Autodesk Inventor part; units mm, degrees
ref_plane "YZ Plane" through (0, 0, 0) normal (1, 0, 0) x (0, 1, 0)
ref_plane "XZ Plane" through (0, 0, 0) normal (0, 1, 0) x (-1, 0, 0)
ref_plane "XY Plane" through (0, 0, 0) normal (0, 0, 1) x (1, 0, 0)
sketch "Sketch1" plane through (0, 0, 0) normal (1, 0, 0) x (0, 1, 0)
  line L0 (0, 0) -> (-25.4, 0)
  line L1 (-25.4, 0) -> (-25.4, -25.4)
  line L2 (-25.4, -25.4) -> (0, -25.4)
  line L3 (0, -25.4) -> (0, 0)
  line L4 (-3.175, -22.225) -> (-22.225, -22.225)
  line L5 (-22.225, -22.225) -> (-22.225, -3.175)
  line L6 (-22.225, -3.175) -> (-3.175, -3.175)
  line L7 (-3.175, -3.175) -> (-3.175, -22.225)
  dimension "d0" = 25.4
  dimension "d1" = 25.4
  dimension "d2" = 3.175
extrude "Extrusion1" add sketch "Sketch1" along normal blind 50.8
sketch "Sketch2" plane through (0, -25.4, 0) normal (0, 0, 1) x (1, 0, 0)
  circle A0 centre (25.4, 12.7) radius 4.7625
  line L0 (0, 25.4) -> (50.8, 25.4)
  line L1 (0, 25.4) -> (0, 0)
  dimension "d5" = 9.525
  dimension "d6" = 12.7
  dimension "d7" = 25.4
extrude "Extrusion2" cut sketch "Sketch2" against normal blind 50.8
sketch "Sketch3" plane through (0, 0, 0) normal (0, 1, 0) x (1, 0, 0)
  circle A0 centre (41.275, 12.7) radius 3.175
  circle A1 centre (9.525, 12.7) radius 3.175
  line L0 (50.8, 25.4) -> (50.8, 0)
  line L1 (0, 25.4) -> (50.8, 25.4)
  line L2 (0, 22.225) -> (0, 3.175)
  point P0 (0, 0)
  dimension "d10" = 6.35
  dimension "d11" = 6.35
  dimension "d12" = 9.525
  dimension "d13" = 12.7
  dimension "d14" = 9.525
  dimension "d15" = 12.7
extrude "Extrusion3" cut sketch "Sketch3" against normal blind 3.175
sketch "Sketch4" plane through (0, -25.4, -25.4) normal (0, -1, 0) x (1, 0, 0)
  circle A0 centre (41.275, 12.7) radius 3.175
  circle A1 centre (41.275, 12.7) radius 4.7625
  circle A2 centre (9.525, 12.7) radius 4.7625
  line L0 (0, 25.4) -> (0, 0)
  line L1 (0, 0) -> (50.8, 0)
  dimension "d18" = 9.525
  dimension "d19" = 9.525
  dimension "d20" = 9.525
  dimension "d21" = 12.7
extrude "Extrusion4" cut sketch "Sketch4" against normal blind 3.175 contours A0 | A1 | A2
properties part number "15102898-16-A-0202" material "Aluminum 6061"
Verification items for the finished model (mm, model axes). A direction names the side the tool comes from. Round coordinates to 2 decimals unless told otherwise and drop trailing zeros. Write each loop counter-clockwise with the first axis right and the second up, starting at its lowest first coordinate (ties: lowest second). Pieces come first, ordered by that corner, then holes. Notation, with made-up numbers: (80.5, 16.25) - (99.5, 16.25) arc R9 cw to (99.5, 20.25) - close; hole circle Ø9 at (-26.5, -10). An arc over 180 degrees is marked (long way). Answer as a JSON object with one key per item and string values. Group by question number.
Q1. Section check D-D, the plane x = 34. Enter the section's corners in (y, z) (3 decimals).
Q2. Go/stop test with a flat-tipped pin: pin 1 Ø8.5 at (x, z) = (41.275, -12.7) entering from -Y (3 decimals). Record where the tip stops, or that it passes through.
Q3. Section check B-B, the plane x = 25.4. Enter the section's corners in (y, z) (1 decimal), plus the area to 3 significant figures.
Q4. Tool access check on faces 1 (the cylindrical face through (36.517, -23.835, -12.491)), 2 (the cylindrical face through (38.1, -1.6, -12.8)), 3 (the flat face through (25, -22.225, -13)). Record the directions out of +Z, -Z, +X, -X, +Y, -Y that give a thin tool (end or side, any length) a straight path to the whole face; none if there is none.
Q5. Mould release check, pull along X, two halves, no side actions. Record for faces 4 (the cylindrical face through (27.96, -8.684, -23.79)), 5 (the cylindrical face through (27.96, -8.684, -1.565)), 6 (the flat face through (25, 0, -13)), 7 (the flat face through (50.8, -2, -13)): released by +X, released by -X, zero draft, split by the parting line, or undercut.
Q6. Section check A-A, the plane z = -5.5. Enter the section's corners in (x, y) (3 decimals), plus the area to 3 significant figures.
Q7. Section check C-C, the plane y = -12.7. Enter the section's corners in (x, z) (1 decimal), plus the area to 3 significant figures.
Q8. Thickness scan on line 1 (Z direction, x = 34.5, y = -15.75) (3 decimals); line 2 (X direction, y = -1.4, z = -12.7). Record the ranges inside material, lowest first.
Found:
{
 "1": {"outline": "(-25.4, -25.4) - (0, -25.4) - (0, 0) - (-25.4, 0) - close; hole (-22.225, -22.225) - (-3.175, -22.225) - (-3.175, -3.175) - (-22.225, -3.175) - close"},
 "2": {"pin 1": "stops at y = -3.175"},
 "3": {"outline": "(-25.4, -25.4) - (-17.5, -25.4) - (-17.5, -22.2) - (-22.2, -22.2) - (-22.2, -3.2) - (-17.5, -3.2) - (-17.5, 0) - (-25.4, 0) - close; (-7.9, -25.4) - (0, -25.4) - (0, 0) - (-7.9, 0) - (-7.9, -3.2) - (-3.2, -3.2) - (-3.2, -22.2) - (-7.9, -22.2) - close", "area": "222 mm^2"},
 "4": {"face 1": "-Y", "face 2": "+Y, -Y", "face 3": "+X, -X"},
 "5": {"face 4": "undercut", "face 5": "undercut", "face 6": "zero draft", "face 7": "released by +X"},
 "6": {"outline": "(0, -25.4) - (50.8, -25.4) - (50.8, -22.225) - (0, -22.225) - close; (0, -3.175) - (50.8, -3.175) - (50.8, 0) - (0, 0) - close", "area": "323 mm^2"},
 "7": {"outline": "(0, -25.4) - (20.6, -25.4) - (20.6, -22.2) - (0, -22.2) - close; (0, -3.2) - (20.6, -3.2) - (20.6, 0) - (0, 0) - close; (30.2, -25.4) - (50.8, -25.4) - (50.8, -22.2) - (30.2, -22.2) - close; (30.2, -3.2) - (50.8, -3.2) - (50.8, 0) - (30.2, 0) - close", "area": "262 mm^2"},
 "8": {"line 1": "z = -25.4 to -22.225, -3.175 to 0", "line 2": "x = 0 to 6.35, 12.7 to 38.1, 44.45 to 50.8"}
}
